Design review of the part built by this model. Coordinates are the model's own, in mm. Face numbers are marked on the shaded views. A direction names the side the tool comes from. Coordinates: 2 decimals unless noted, no trailing zeros. Loops run counter-clockwise (first coordinate to the right, second up) from the corner with the lowest first, then second, coordinate; pieces in that order, holes last.
Q1. Add section B-B on z = -64.5. Give the boundary of the cut face in (x, y), and give its area (3 significant figures).
Q2. Add section D-D on y = -3. Give the boundary of the cut face in (x, z), and give its area (3 significant figures).
Q3. Wall thickness on probe 1 along X at (y, z) = (12, -95); probe 2 along Z at (x, y) = (34, 32.5); probe 3 along Y at (x, z) = (94.5, -76): over which ranges is each line inside the solid? List them lowest first.
Q4. For P1, Ø8, axis at y = -9, z = -18.5, coming from the -X side; P2, Ø12, axis at y = -18.5, z = -117, coming from the +X side, all flat-tipped, find the tip position at first contact; note any pin that passes through.
Q5. Draft analysis for pull direction X (two halves, no side actions). For the marked faces 1, 2, 3 and 4, state which applies: released by +X, released by -X, zero draft, split by the parting line, or undercut.
Q6. Add section A-A on x = 63.5. Give the boundary of the cut face in (y, z).
Q7. Add section C-C on y = 17.5. Give the boundary of the cut face in (x, z).
Q8. Machinability: for the marked faces 5 and 6, which of the approach directions +Z, -Z, +X, -X, +Y, -Y give a long, thin tool a straight path to every point of the face, cutting with its end or side? Answer none if there is none.
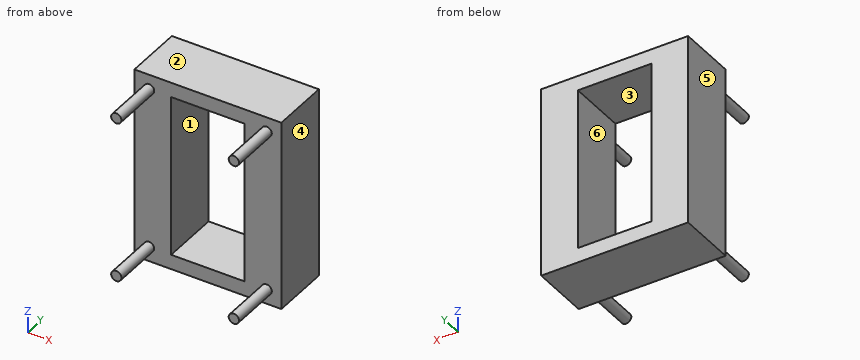
Autodesk Inventor part; units mm, degrees
ref_plane "YZ Plane" through (0, 0, 0) normal (1, 0, 0) x (0, 1, 0)
ref_plane "XZ Plane" through (0, 0, 0) normal (0, 1, 0) x (-1, 0, 0)
ref_plane "XY Plane" through (0, 0, 0) normal (0, 0, 1) x (1, 0, 0)
sketch "Sketch1" plane through (0, 0, 0) normal (0, 1, 0) x (-1, 0, 0)
  line L0 (0, 0) -> (-100, 0)
  line L1 (-100, 0) -> (-100, -130)
  line L2 (-100, -130) -> (0, -130)
  line L3 (0, -130) -> (0, 0)
  dimension "d0" = 100
  dimension "d1" = 130
extrude "Extrusion1" add sketch "Sketch1" along normal blind 40
sketch "Sketch2" plane through (0, 40, 0) normal (0, 1, 0) x (1, 0, 0)
  line L0 (25, 10) -> (75, 10)
  line L1 (75, 10) -> (75, 120)
  line L2 (75, 120) -> (25, 120)
  line L3 (25, 120) -> (25, 10)
  line L4 (100, 130) -> (0, 130)
  line L5 (0, 0) -> (100, 0)
  line L6 (0, 130) -> (0, 0)
  line L7 (100, 0) -> (100, 130)
  dimension "d4" = 10
  dimension "d5" = 10
  dimension "d6" = 25
  dimension "d7" = 25
extrude "Extrusion2" cut sketch "Sketch2" against normal blind 40 contours L3 L2 L1 L0
sketch "Sketch3" plane through (0, 0, 0) normal (0, -1, 0) x (1, 0, 0)
  circle A0 centre (90, -10) radius 3.5
  line L0 (100, 0) -> (100, -130)
  line L1 (0, 0) -> (100, 0)
  line L2 (0, 0) -> (100, 0)
  line L3 (50, 0) -> (50, -130)
  line L4 (100, 0) -> (100, -130)
  line L5 (100, -65) -> (0, -65)
  line L6 (0, -130) -> (0, 0)
  circle A1 centre (90, -120) radius 3.5
  circle A2 centre (10, -10) radius 3.5
  line L7 (0, 0) -> (0, -130)
  line L8 (0, 0) -> (0, -130)
  circle A3 centre (10, -120) radius 3.5
  dimension "d10" = 7
  dimension "d11" = 10
  dimension "d12" = 10
extrude "Extrusion3" add sketch "Sketch3" along normal blind 35 contours A0 | A1 | A2 | A3
properties part number "top"
Entries:
1. outline: (0, 0) - (25, 0) - (25, 40) - (0, 40) - close; (75, 0) - (100, 0) - (100, 40) - (75, 40) - close
1. area: 2,000 mm2
2. outline: circle Ø7 at (10, -120); circle Ø7 at (10, -10); circle Ø7 at (90, -120); circle Ø7 at (90, -10)
2. area: 154 mm2
3. probe 1: x = 0 to 25, 75 to 100
3. probe 2: z = -130 to -120, -10 to 0
3. probe 3: y = 0 to 40
4. P1: passes through
4. P2: stops at x = 93.5
5. face 1: undercut
5. face 2: zero draft
5. face 3: undercut
5. face 4: released by +X
6. outline: (0, -130) - (40, -130) - (40, -120) - (0, -120) - close; (0, -10) - (40, -10) - (40, 0) - (0, 0) - close
7. outline: (0, -130) - (100, -130) - (100, 0) - (0, 0) - close; hole (25, -120) - (75, -120) - (75, -10) - (25, -10) - close
8. face 5: +Z, -Z, -X, +Y, -Y
8. face 6: +Y, -Y
